Source: three-view drawing plus pictorial views. Frame: mm from the lowest corner of the part. Coordinates: 2 decimals unless noted, no trailing zeros. Write each loop counter-clockwise with the first axis right and the second up, starting at its lowest first coordinate (ties: lowest second). Pieces come first, ordered by that corner, then holes.
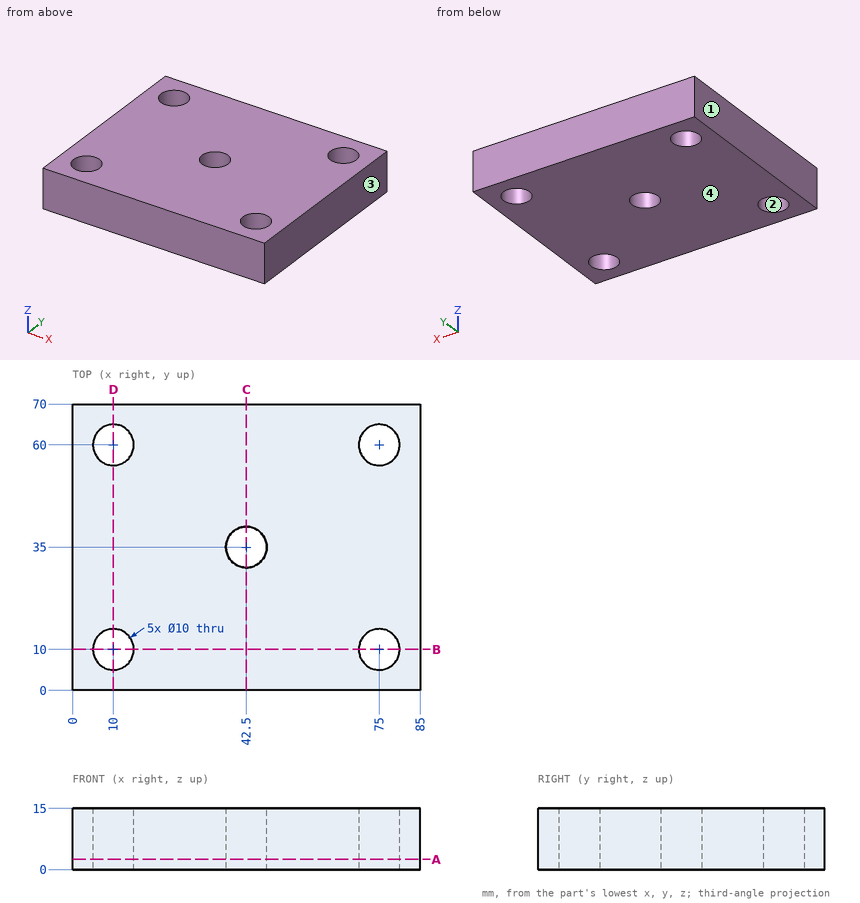
Item 1: Section query A-A, the plane z = 2.5. Return loops of the section in (x, y), then the cut area to 3 significant figures.
Item 2: Material intervals for line 1 (Y direction, x = 10, z = 5.5); line 2 (Y direction, x = 8, z = 1.25); line 3 (Y direction, x = 42.5, z = 6.5), sorted ascending.
Item 3: Section query C-C, the plane x = 42.5. Return loops of the section in (y, z).
Item 4: Pin query (flat end, axial travel): pin 1 Ø6 at (x, z) = (14.5, 7.5) entering from -Y; pin 2 Ø9 at (x, y) = (75, 10) entering from -Z. Return the tip coordinate at first contact, or that it passes through.
Item 5: Pull-direction query (X, two-part tool) for the marked faces 1, 2, 3 and 4; classes: released by +X, released by -X, zero draft, split by the parting line, or undercut.
Item 6: Section query B-B, the plane y = 10. Return loops of the section in (x, z).
Item 7: Section query D-D, the plane x = 10. Return loops of the section in (y, z), then the cut area to 3 significant figures.
The answers:
1. outline: (0, 0) - (85, 0) - (85, 70) - (0, 70) - close; hole circle Ø10 at (10, 10); hole circle Ø10 at (10, 60); hole circle Ø10 at (42.5, 35); hole circle Ø10 at (75, 10); hole circle Ø10 at (75, 60)
1. area: 5,560 mm2
2. line 1: y = 0 to 5, 15 to 55, 65 to 70
2. line 2: y = 0 to 5.42, 14.58 to 55.42, 64.58 to 70
2. line 3: y = 0 to 30, 40 to 70
3. outline: (0, 0) - (30, 0) - (30, 15) - (0, 15) - close; (40, 0) - (70, 0) - (70, 15) - (40, 15) - close
4. pin 1: stops at y = 0
4. pin 2: passes through
5. face 1: released by -X
5. face 2: undercut
5. face 3: released by +X
5. face 4: zero draft
6. outline: (0, 0) - (5, 0) - (5, 15) - (0, 15) - close; (15, 0) - (70, 0) - (70, 15) - (15, 15) - close; (80, 0) - (85, 0) - (85, 15) - (80, 15) - close
7. outline: (0, 0) - (5, 0) - (5, 15) - (0, 15) - close; (15, 0) - (55, 0) - (55, 15) - (15, 15) - close; (65, 0) - (70, 0) - (70, 15) - (65, 15) - close
7. area: 750 mm2
